Build history of the part. All positions in model axes, mm. A direction names the side the tool comes from. Give positions to 0.01 mm unless a question says otherwise; leave off trailing zeros. Order: outer loops, then holes, each group sorted by start corner. A loop starts at its lowest first (then second) coordinate and runs counter-clockwise, first axis right, second up. Notation, with made-up numbers: (88, 40) - (102, 40) arc R15 ccw to (102, 46) - close; hole circle Ø8 at (1, 71). An arc over 180 degrees is marked (long way). One line per item, written item: value.
```python
from build123d import *

# Parameters (mm, degrees)
SKETCH1_W               = 325.28
SKETCH1_H               = 30
BOSS_EXTRUDE1_DEPTH     = 3
SKETCH2_W               = 3
SKETCH2_H               = 15
CUT_EXTRUDE1_DEPTH      = 1
CUT_EXTRUDE1_DEPTH_BACK = 4
CUT_EXTRUDE3_DEPTH      = 4


with BuildPart() as part:
    # Sketch1 → Boss-Extrude1 (new body)
    with BuildSketch(Plane(origin=(0, 0, 0), x_dir=(1, 0, 0), z_dir=(0, 1, 0))):
        with Locations((162.64, 0)):
            Rectangle(SKETCH1_W, SKETCH1_H)
    extrude(amount=BOSS_EXTRUDE1_DEPTH)

    # Sketch2 → Cut-Extrude1 (cut, two sides)
    with BuildSketch(Plane(origin=(0, 3, 0), x_dir=(1, 0, 0), z_dir=(0, 1, 0))) as cut_extrude1_sk:
        with Locations((81.5, -7.5)):
            Rectangle(SKETCH2_W, SKETCH2_H)
        with Locations((208.4, -7.5)):
            Rectangle(SKETCH2_W, SKETCH2_H)
    extrude(amount=CUT_EXTRUDE1_DEPTH, mode=Mode.SUBTRACT)
    extrude(cut_extrude1_sk.sketch, amount=-CUT_EXTRUDE1_DEPTH_BACK, mode=Mode.SUBTRACT)

    # Sketch4 → Cut-Extrude3 (cut, through all)
    with BuildSketch(Plane(origin=(0, 3, 0), x_dir=(1, 0, 0), z_dir=(0, 1, 0))):
        with BuildLine():
            Line((15, 9), (65, 9))
            ThreePointArc((65, 9), (74, 0), (65, -9))
            Line((65, -9), (15, -9))
            ThreePointArc((15, -9), (6, 0), (15, 9))
        make_face()
        with BuildLine():
            Line((98, 9), (191.9, 9))
            ThreePointArc((191.9, 9), (200.9, 0), (191.9, -9))
            Line((191.9, -9), (98, -9))
            ThreePointArc((98, -9), (89, 0), (98, 9))
        make_face()
        with BuildLine():
            Line((224.9, 9), (295.28, 9))
            ThreePointArc((295.28, 9), (304.28, 0), (295.28, -9))
            Line((295.28, -9), (224.9, -9))
            ThreePointArc((224.9, -9), (215.9, 0), (224.9, 9))
        make_face()
    extrude(amount=-CUT_EXTRUDE3_DEPTH, mode=Mode.SUBTRACT)


solid = part.part
```
(1) Drill centre lines: line 1 (X direction, y = 2.1, z = 10.5); line 2 (Z direction, x = 190.5, y = 2.9); line 3 (X direction, y = 1.9, z = -8). Where is each one in solid material? Low to high.
Completed:
line 1: 0 to 80, 83 to 206.9, 209.9 to 325.28
line 2: -15 to -9, 9 to 15
line 3: 0 to 10.88, 69.12 to 93.88, 196.02 to 220.78, 299.4 to 325.28
(2) Slice it at A-A, the plane y = 1.8. Give the cut face in (x, z), and give its area (3 significant figures).
Completed:
outline: (0, -15) - (325.28, -15) - (325.28, 15) - (209.9, 15) - (209.9, 0) - (206.9, 0) - (206.9, 15) - (83, 15) - (83, 0) - (80, 0) - (80, 15) - (0, 15) - close; hole (15, -9) - (65, -9) arc R9 ccw to (65, 9) - (15, 9) arc R9 ccw to start; hole (98, -9) - (191.9, -9) arc R9 ccw to (191.9, 9) - (98, 9) arc R9 ccw to start; hole (224.9, -9) - (295.28, -9) arc R9 ccw to (295.28, 9) - (224.9, 9) arc R9 ccw to start
area: 5,050 mm²
(3) 3-axis set-ups, long thin cutter, end or side, ignore diameter. For faces 1 (the face through (304.278, 1.521, -0.198)), 2 (the face through (160, 0, -10)): which of +Z, -Z, +X, -X, +Y, -Y reach the whole face in a straight line?
Completed:
face 1: +Y, -Y
face 2: +Z, -Z, +X, -X, -Y
(4) Pin check, flat tips, straight feed: P1, Ø6, axis at x = 95, z = 2, coming from the +Y side; P2, Ø1.5, axis at x = 81.5, y = 1, coming from the +Z side. Stop position of each tip, or through.
Completed:
P1: through
P2: z = 0
(5) Slice it at B-B, the plane x = 52.5. Give the cut face in (y, z), and give its area (3 significant figures).
Completed:
outline: (0, -15) - (3, -15) - (3, -9) - (0, -9) - close; (0, 9) - (3, 9) - (3, 15) - (0, 15) - close
area: 36.0 mm²
(6) Pull direction Z, two halves, no side cores. Call faces 3 (the face through (89, 2, 0)), 4 (the face through (160, 3, -10)), 5 (the face through (74, 2, 0)): +Z half, -Z half, draft (parallel to the pull), parting line (faces both ways), or undercut.
Completed:
face 3: undercut
face 4: draft
face 5: undercut
